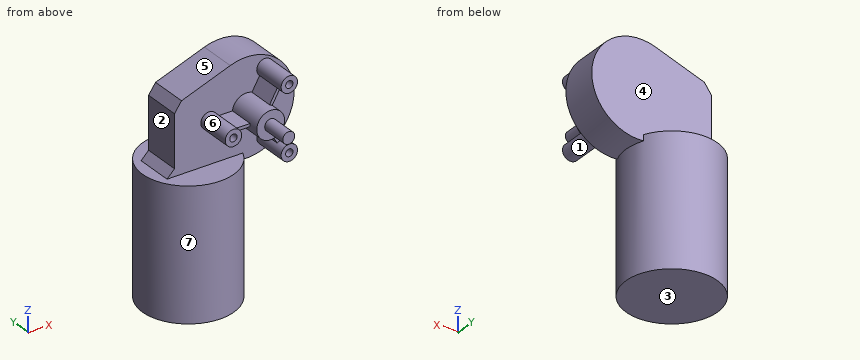
Solid Edge part; units mm, degrees
sketch "Sketch1" plane through (0, 0, 0) normal (0, -1, 0) x (1, 0, 0)
  line L0 (-16.1, 16.9) -> (-16.1, -29.1)
  line L1 (18.5501, -29.1) -> (-16.1, -29.1)
  line L2 (-16.1, 16.9) -> (21.324, 30.2372)
  arc A0 (18.5501, -29.1) -> (21.324, 30.2372) centre (32.1, 0) ccw
  dimension "D1" = 16.1
  dimension "D2" = 16.1
extrude "Extrusionsausprägung_1" add sketch "Sketch1" against normal blind 12.5 and the other way blind 12.5
sketch "Sketch2" plane through (24.05, -12.5, 0) normal (0, -1, 0) x (1, 0, 0)
  circle A0 centre (8.05, 0) radius 9.35
  circle A1 centre (20.55, 21.6506) radius 5.5
  circle A2 centre (20.55, -21.6506) radius 5.5
  circle A3 centre (-16.95, 0) radius 5.5
extrude "Extrusionsausprägung_2" add sketch "Sketch2" along normal blind 23.5
sketch "Sketch3" plane through (32.1, -36, 0) normal (0, -1, 0) x (1, 0, 0)
  circle A0 centre (0, 0) radius 4
extrude "Extrusionsausprägung_3" add sketch "Sketch3" along normal blind 17.4
sketch "Sketch4" plane through (24.05, -12.5, 0) normal (0, -1, 0) x (1, 0, 0)
  line L0 (-11.5417, 1) -> (-1.2464, 1)
  line L1 (-11.5417, -1) -> (-1.2464, -1)
  arc A0 (-11.5417, -1) -> (-11.5417, 1) centre (-16.95, 0) ccw
  arc A1 (-1.2464, 1) -> (-1.2464, -1) centre (8.05, 0) ccw
extrude "Extrusionsausprägung_4" add sketch "Sketch4" along normal blind 17
pattern_circular "Pattern1" count 3 over 360 about axis through (32.1, -12.5, 0) along (0, 1, 0) of "Extrusionsausprägung_4"
cosmetic_thread "Thread1"
hole "Bohrung_1" at (7.1, -36, 0) direction (0, 1, 0) diameter 4.917 depth 10 tip angle 118 thread major 6 thread length 8
hole "Hole1" at (44.6, -36, 21.6506) direction (0, 1, 0) diameter 4.917 depth 10 tip angle 118 thread major 6 thread length 8
hole "Hole2" at (44.6, -36, -21.6506) direction (0, 1, 0) diameter 4.917 depth 10 tip angle 118 thread major 6 thread length 8
sketch "Sketch5" plane through (0, 0, -28) normal (0, 0, 1) x (1, 0, 0)
  circle A0 centre (1.6, -0.3) radius 30.7
extrude "Extrusionsausprägung_7" add sketch "Sketch5" against normal blind 87.5
chamfer "Fase_1" distance 5 angle 45 1 edges at (-16.1, 0, 16.9)
chamfer "Fase_2" distance 5 angle 45 1 edges at (-16.1, 0, -28)
Read the model definition and answer for the solid it produces. Units are mm, in the model's axes. Face numbers are marked on the shaded views. A direction names the side the tool comes from. Round coordinates to 2 decimals unless told otherwise and drop trailing zeros. Loops run counter-clockwise (first coordinate to the right, second up) from the corner with the lowest first, then second, coordinate; pieces in that order, holes last.
Q1. Section C-C on x = 34 is taken. Write down the section's boundary in (y, z), and give its area (3 significant figures).
Q2. Each of these flat-tipped pins is pushed along its axis until it touches: pin 1 (12 mm diameter, centred on x = 9, z = -2, fed in from -Y); pin 2 (7.5 mm diameter, centred on x = 40, z = 13, fed in from -Y); pin 3 (6 mm diameter, centred on x = 16, y = -34, fed in from +Z); pin 4 (4 mm diameter, centred on x = 44.6, z = -21.65, fed in from -Y). Where does it stop, or does it pass through?
Q3. Which of the six approach directions +Z, -Z, +X, -X, +Y, -Y give full straight-line access (tool end or side, diameter ignored) to the marked faces 1, 2 and 3?
Q4. Section B-B on z = -85 is taken. Write down the section's boundary in (x, y).
Q5. Determine the mould class of the marked faces 4, 5, 6 and 7 for opening direction X: released by +X, released by -X, zero draft, split by the parting line, or undercut.
Q6. Consider probe 1 along Z at (x, y) = (44.6, -30.5); probe 2 along Z at (x, y) = (44, -31); probe 3 along Z at (x, y) = (7, -33). Determine where each line is inside the solid, lowest interval first.
Q7. Section D-D on y = -42 is taken. Write down the section's boundary in (x, z), and give its area (3 significant figures).
Q8. Section A-A on y = -0.3 is taken. Write down the section's boundary in (x, z), and give its area (3 significant figures).
Output:
1. outline: (-53.4, -3.52) - (-36, -3.52) - (-36, -9.15) - (-12.5, -9.15) - (-12.5, -32.04) - (12.5, -32.04) - (12.5, 32.04) - (-12.5, 32.04) - (-12.5, 9.15) - (-36, 9.15) - (-36, 3.52) - (-53.4, 3.52) - close
1. area: 2,150 mm2
2. pin 1: stops at y = -36
2. pin 2: stops at y = -29.5
2. pin 3: passes through
2. pin 4: stops at y = -25.72
3. face 1: -Y
3. face 2: +Z, -X, +Y, -Y
3. face 3: -Z, +X, -X, +Y, -Y
4. outline: circle Ø61.4 at (1.6, -0.3)
5. face 4: zero draft
5. face 5: released by -X
5. face 6: undercut
5. face 7: split by the parting line
6. probe 1: z = -27.15 to -24.11, -19.19 to -16.15, 16.15 to 19.19, 24.11 to 27.15
6. probe 2: z = -27.12 to -24.03, -19.27 to -16.18, 16.18 to 19.27, 24.03 to 27.12
6. probe 3: z = -5.5 to -2.46, 2.46 to 5.5
7. outline: circle Ø8 at (32.1, 0)
7. area: 50.3 mm2
8. outline: (-29.1, -115.5) - (32.3, -115.5) - (32.3, -32.1) arc R32.1 ccw (long way) to (21.32, 30.24) - (-11.39, 18.58) - (-16.1, 11.9) - (-16.1, -23) - (-21.1, -28) - (-29.1, -28) - close
8. area: 9,560 mm2
